Geometry: final body of the model. Coordinates: model frame, mm. A direction names the side the tool comes from. Round coordinates to 2 decimals unless told otherwise and drop trailing zeros. Write each loop counter-clockwise with the first axis right and the second up, starting at its lowest first coordinate (ties: lowest second). Pieces come first, ordered by that corner, then holes. Notation, with made-up numbers: (-23.75, 60) - (30.25, 60) arc R22 ccw to (30.25, 94) - close; hole circle Ø4 at (-18, -14.5). An arc over 180 degrees is marked (long way). Write each question's results on one line, items separated by ' | '.
from build123d import *

# Parameters (mm, degrees)
BASE_EXTRUDE_DEPTH       = 16.637
SKETCH2_R                = 4.1656
HOLE1_DEPTH              = 110.03976233
HOLE1_PATTERN_COUNT      = 2
HOLE1_PATTERN_PITCH      = 38.1
HOLE1_PATTERN_COUNT_DIR2 = 2
HOLE1_PATTERN_PITCH_DIR2 = 38.1
SKETCH3_R                = 4.1656
HOLE2_DEPTH              = 110.03976233
HOLE2_PATTERN_COUNT      = 2
HOLE2_PATTERN_PITCH      = 38.1
HOLE2_PATTERN_COUNT_DIR2 = 2
HOLE2_PATTERN_PITCH_DIR2 = 38.1


with BuildPart() as part:
    # Sketch1 → Base Extrude (new, symmetric)
    with BuildSketch(Plane(origin=(0, 0, 0), x_dir=(0, 0, -1), z_dir=(1, 0, 0))):
        with BuildLine():
            Line((-6.35, 12.7), (-6.35, 69.85))
            ThreePointArc((-6.35, 69.85), (-4.490128061, 74.340128061), (0, 76.2))
            Line((0, 76.2), (0, 0))
            Line((0, 0), (-76.2, 0))
            ThreePointArc((-76.2, 0), (-74.340128061, 4.490128061), (-69.85, 6.35))
            Line((-69.85, 6.35), (-12.7, 6.35))
            ThreePointArc((-12.7, 6.35), (-8.209871939, 8.209871939), (-6.35, 12.7))
        make_face()
    extrude(amount=BASE_EXTRUDE_DEPTH, both=True)

    # Sketch2 → Hole1 (cut, through all)
    with BuildSketch(Plane.XZ):
        with Locations(Location((0, 19.05, 0), (0, 0, 270))):
            Circle(SKETCH2_R)
    hole1 = extrude(amount=-HOLE1_DEPTH, mode=Mode.SUBTRACT)

    # Hole1 Pattern: Hole1 2 × 2
    with Locations(*[(i * HOLE1_PATTERN_PITCH, 0, j * HOLE1_PATTERN_PITCH_DIR2) for i in range(HOLE1_PATTERN_COUNT) for j in range(HOLE1_PATTERN_COUNT_DIR2) if (i, j) != (0, 0)]):
        add(hole1, mode=Mode.SUBTRACT)

    # Sketch3 → Hole2 (cut, through all)
    with BuildSketch(Plane(origin=(0, 0, 0), x_dir=(-1, 0, 0), z_dir=(0, 0, -1))):
        with Locations(Location((0, 19.05, 0), (0, 0, 90))):
            Circle(SKETCH3_R)
    hole2 = extrude(amount=-HOLE2_DEPTH, mode=Mode.SUBTRACT)

    # Hole2 Pattern: Hole2 2 × 2
    with Locations(*[(i * HOLE2_PATTERN_PITCH, j * HOLE2_PATTERN_PITCH_DIR2, 0) for i in range(HOLE2_PATTERN_COUNT) for j in range(HOLE2_PATTERN_COUNT_DIR2) if (i, j) != (0, 0)]):
        add(hole2, mode=Mode.SUBTRACT)


solid = part.part
Q1. Ray query, line 1 along Z through (x, y) = (-3.5, 49); line 2 along X through (y, z) = (1, 19). Return the intervals inside material, ascending.
Answer block:
line 1: 0 to 6.35 | line 2: -16.64 to -4.17, 4.17 to 16.64
Q2. Access query for faces 5 (the cylindrical face through (2.815, 3.131, 60.22)), 6 (the flat face through (0, 6.35, 42)). Directions: +Z, -Z, +X, -X, +Y, -Y. A direction counts if a zero-diameter tool reaches every point of the face in a straight line with its end or side. Return the directions, or none.
Answer block:
face 5: +Y, -Y | face 6: +Z, +X, -X, +Y
Q3. Pin query (flat end, axial travel): pin 1 (7.5 mm diameter, centred on x = 0, z = 19.05, fed in from -Y); pin 2 (11 mm diameter, centred on x = 0, y = 57.15, fed in from +Z); pin 3 (8 mm diameter, centred on x = 9, z = 29.5, fed in from +Y). Return the tip coordinate at first contact, or that it passes through.
Answer block:
pin 1: through | pin 2: z = 6.35 | pin 3: y = 6.35
Q4. Section query C-C, the plane x = 13.5. Return loops of the section in (y, z).
Answer block:
outline: (0, 0) - (76.2, 0) arc R6.35 ccw to (69.85, 6.35) - (12.7, 6.35) arc R6.35 cw to (6.35, 12.7) - (6.35, 69.85) arc R6.35 ccw to (0, 76.2) - close
Q5. Mould query, pull axis X, two halves, no side actions, for faces 1 (the cylindrical face through (0.23, 8.16, 8.26)), 2 (the cylindrical face through (1.251, 23.023, 3.131)), 3 (the flat face through (-16.637, 21, 4)), 4 (the cylindrical face through (1.251, 61.123, 3.131)). Classes: pulls with the +X half, pulls with the -X half, needs draft (parallel to the pull), parting line crosses it, or undercut.
Answer block:
face 1: needs draft | face 2: undercut | face 3: pulls with the -X half | face 4: undercut
Q6. Section query A-A, the plane y = 57.15. Return loops of the section in (x, z), plus the area to 3 significant figures.
Answer block:
outline: (-16.64, 0) - (-4.17, 0) - (-4.17, 6.35) - (-16.64, 6.35) - close; (4.17, 0) - (16.64, 0) - (16.64, 6.35) - (4.17, 6.35) - close | area: 158 mm2
Q7. Section query D-D, the plane z = 29. Return loops of the section in (x, y).
Answer block:
outline: (-16.64, 0) - (16.64, 0) - (16.64, 6.35) - (-16.64, 6.35) - close
